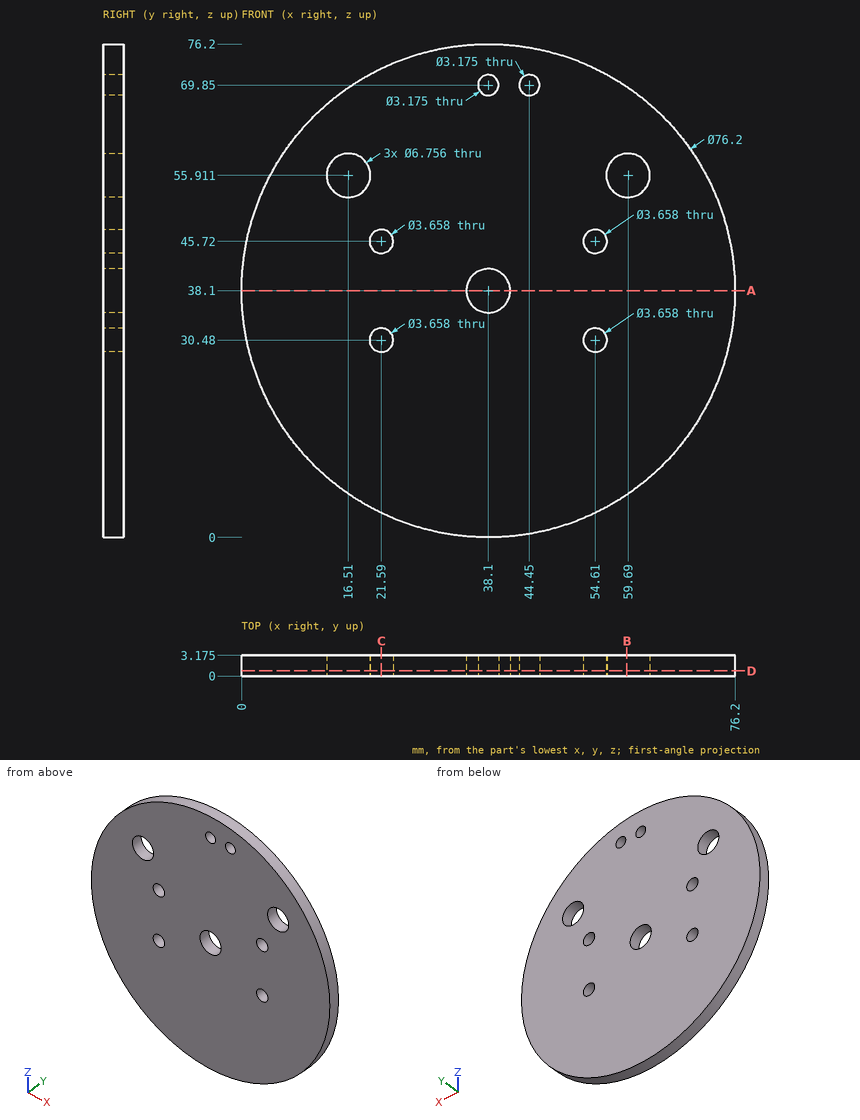
Here's the drawing with two shaded views (mm, measured from the low corner). I have some questions. Give positions to 0.01 mm unless a question says otherwise; leave off trailing zeros. Loops run counter-clockwise (first coordinate to the right, second up) from the corner with the lowest first, then second, coordinate; pieces in that order, holes last. Notation, with made-up numbers: M -35,20 L 8,20 A30 cw 8,45 Z; hole C 14,-33.75 d1. An arc over 180 degrees is marked long. Use one line per item in the form item = value. Start each with the question number.
Q1. If we section it at D-D (y = 0.8): State how many separate pieces and enclosed holes the cut face has, then the cut area to 4 significant figures.
Q2. If we section it at B-B (x = 59.5): Write out the boundary of the cut face in (y, z) (1 decimal), then the cut area to 3 significant figures.
Q3. If we section it at C-C (x = 21.59): Write out the boundary of the cut face in (y, z) (1 decimal), then the cut area to 3 significant figures.
Q4. Will this pin go through, and if not, where does the flat tip stop? pin 1 Ø1 at (y, z) = (2, 51) entering from +X (1 decimal).
Q5. If we section it at A-A (z = 38.1): Write out the boundary of the cut face in (x, y) (1 decimal).
Q6. I need wall thicknesses on line 1 along Z through (x, y) = (38.1, 2.1); line 2 along X through (y, z) = (2.85, 55); line 3 along Z through (x, y) = (54.61, 2.15). Which ranges of each line are inside material? Lowest first, please.
Taken from the geometry:
q1.separate_pieces = 1
q1.enclosed_holes = 9
q1.area = 4,395 mm^2
q2.outline = M 0,6.6 L 3.2,6.6 L 3.2,52.5 L 0,52.5 Z; M 0,59.3 L 3.2,59.3 L 3.2,69.6 L 0,69.6 Z
q2.area = 179 mm^2
q3.outline = M 0,3.8 L 3.2,3.8 L 3.2,28.7 L 0,28.7 Z; M 0,32.3 L 3.2,32.3 L 3.2,43.9 L 0,43.9 Z; M 0,47.5 L 3.2,47.5 L 3.2,72.4 L 0,72.4 Z
q3.area = 195 mm^2
q4.pin_1 = 74.1
q5.outline = M 0,0 L 34.7,0 L 34.7,3.2 L 0,3.2 Z; M 41.5,0 L 76.2,0 L 76.2,3.2 L 41.5,3.2 Z
q6.line_1 = 0 to 34.72, 41.48 to 68.26, 71.44 to 76.2
q6.line_2 = 3.95 to 13.26, 19.76 to 56.44, 62.94 to 72.25
q6.line_3 = 3.76 to 28.65, 32.31 to 43.89, 47.55 to 72.44
